from build123d import *

# Parameters (mm, degrees)
F0_W     = 20
F0_H     = 35
F1_DEPTH = 1.5
F2_R     = 1
F3_DEPTH = 1.5
F4_R     = 3
F5_R     = 10
F6_R     = 1
F7_DEPTH = 2
F8_R     = 1.5
F8_R_2   = 1
F9_DEPTH = 1.5


with BuildPart() as f1:
    # F0 (on Top) → F1 (new body)
    with BuildSketch(Plane.XY):
        Rectangle(F0_W, F0_H)
    extrude(amount=-F1_DEPTH)

    # F2 (on face) → F3 (cut)
    with BuildSketch(Plane.XY):
        with Locations((-8, 15.5)):
            Circle(F2_R)
        with Locations((-8, 7.5)):
            Circle(F2_R)
        with Locations((-8, 0)):
            Circle(F2_R)
        with Locations((-8, -7.5)):
            Circle(F2_R)
        with Locations((-8, -15.5)):
            Circle(F2_R)
    extrude(amount=-F3_DEPTH, mode=Mode.SUBTRACT)

    # F4
    f4_edges = [f1.edges().sort_by_distance(p)[0] for p in [
        (-10, -17.5, -0.75),
        (-10, 17.5, -0.75),
    ]]
    fillet(f4_edges, radius=F4_R)

    # F5
    f5_edges = [f1.edges().sort_by_distance(p)[0] for p in [
        (10, 17.5, -0.75),
        (10, -17.5, -0.75),
    ]]
    fillet(f5_edges, radius=F5_R)

    # F6 (on face) → F7 (join)
    with BuildSketch(Plane.XY):
        Circle(F6_R)
        with Locations((4, 0)):
            Circle(F6_R)
        with Locations((8, 0)):
            Circle(F6_R)
    extrude(amount=F7_DEPTH)

    # F8 (on face) → F9 (join)
    with BuildSketch(Plane.XY.offset(2)):
        Circle(F8_R)
        Circle(F8_R_2, mode=Mode.SUBTRACT)
        with Locations((4, 0)):
            Circle(F8_R)
        with Locations((8, 0)):
            Circle(F8_R)
        Circle(F8_R_2)
    extrude(amount=F9_DEPTH)


solid = f1.part
The listing builds one solid part. Answer for the finished solid, in the listing's coordinates (mm). A direction names the side the tool comes from. Coordinates: 2 decimals unless noted, no trailing zeros. Loops run counter-clockwise (first coordinate to the right, second up) from the corner with the lowest first, then second, coordinate; pieces in that order, holes last. Notation, with made-up numbers: (87.25, 69.5) -> (143.25, 69.5) arc R27 ccw to (143.25, 101.5) -> close; hole circle Ø5 at (51, -14). An arc over 180 degrees is marked (long way). Answer in a Markdown table with one row per item. Add a question column.
1. The part is cut by section C-C, the plane x = -8. Write down the section's boundary in (y, z), then the cut area to 3 significant figures.
2. Flat-ended cylindrical pins translate along their axes: P1, Ø1.2, axis at x = -8, y = 7.5, coming from the +Z side; P2, Ø5, axis at x = -7, y = 4.5, coming from the +Z side. Find the tip coordinate at first contact, or state that the pin passes through.
3. The part is cut by section B-B, the plane z = -1. Write down the section's boundary in (x, y).
4. Consider line 1 (Y direction, x = -8, z = -0.3); line 2 (Z direction, x = 7.75, y = 5.5); line 3 (X direction, y = -0.5, z = -0.8). Determine where each line is inside the solid, lowest interval first. Write a range as [from, to].
5. The part is cut by section D-D, the plane x = 8. Write down the section's boundary in (y, z).
6. For faces 1 (the cylindrical face through (5.386, -0.575, 2.74)), 2 (the cylindrical face through (-9.14, -16.6, -0.76)), determine the directions among +Z, -Z, +X, -X, +Y, -Y from which every point of the face is accessible in a straight line to the end or side of a thin tool.
7. Determine the mould class of faces 3 (the cylindrical face through (3, 0, 1)), 4 (the flat face through (8, 0, 3.5)), 5 (the flat face through (0, 0, -1.5)), 6 (the cylindrical face through (-8.217, 14.524, -0.74)) for opening direction Z: +Z half, -Z half, draft (parallel to the pull), parting line (faces both ways), or undercut.
Answer below:
| question | item | result |
|---|---|---|
| 1 | outline | (-17.33, -1.5) -> (-16.5, -1.5) -> (-16.5, 0) -> (-17.33, 0) -> close; (-14.5, -1.5) -> (-8.5, -1.5) -> (-8.5, 0) -> (-14.5, 0) -> close; (-6.5, -1.5) -> (-1, -1.5) -> (-1, 0) -> (-6.5, 0) -> close; (1, -1.5) -> (6.5, -1.5) -> (6.5, 0) -> (1, 0) -> close; (8.5, -1.5) -> (14.5, -1.5) -> (14.5, 0) -> (8.5, 0) -> close; (16.5, -1.5) -> (17.33, -1.5) -> (17.33, 0) -> (16.5, 0) -> close |
| 1 | area | 37.0 mm2 |
| 2 | P1 | through |
| 2 | P2 | z = 0 |
| 3 | outline | (-10, -14.5) arc R3 ccw to (-7, -17.5) -> (0, -17.5) arc R10 ccw to (10, -7.5) -> (10, 7.5) arc R10 ccw to (0, 17.5) -> (-7, 17.5) arc R3 ccw to (-10, 14.5) -> close; hole circle Ø2 at (-8, -15.5); hole circle Ø2 at (-8, -7.5); hole circle Ø2 at (-8, 0); hole circle Ø2 at (-8, 7.5); hole circle Ø2 at (-8, 15.5) |
| 4 | line 1 | [-17.33, -16.5], [-14.5, -8.5], [-6.5, -1], [1, 6.5], [8.5, 14.5], [16.5, 17.33] |
| 4 | line 2 | [-1.5, 0] |
| 4 | line 3 | [-10, -8.87], [-7.13, 10] |
| 5 | outline | (-13.5, -1.5) -> (13.5, -1.5) -> (13.5, 0) -> (1, 0) -> (1, 2) -> (1.5, 2) -> (1.5, 3.5) -> (-1.5, 3.5) -> (-1.5, 2) -> (-1, 2) -> (-1, 0) -> (-13.5, 0) -> close |
| 6 | face 1 | +Z |
| 6 | face 2 | +Z, -Z, -X, -Y |
| 7 | face 3 | undercut |
| 7 | face 4 | +Z half |
| 7 | face 5 | -Z half |
| 7 | face 6 | draft |
